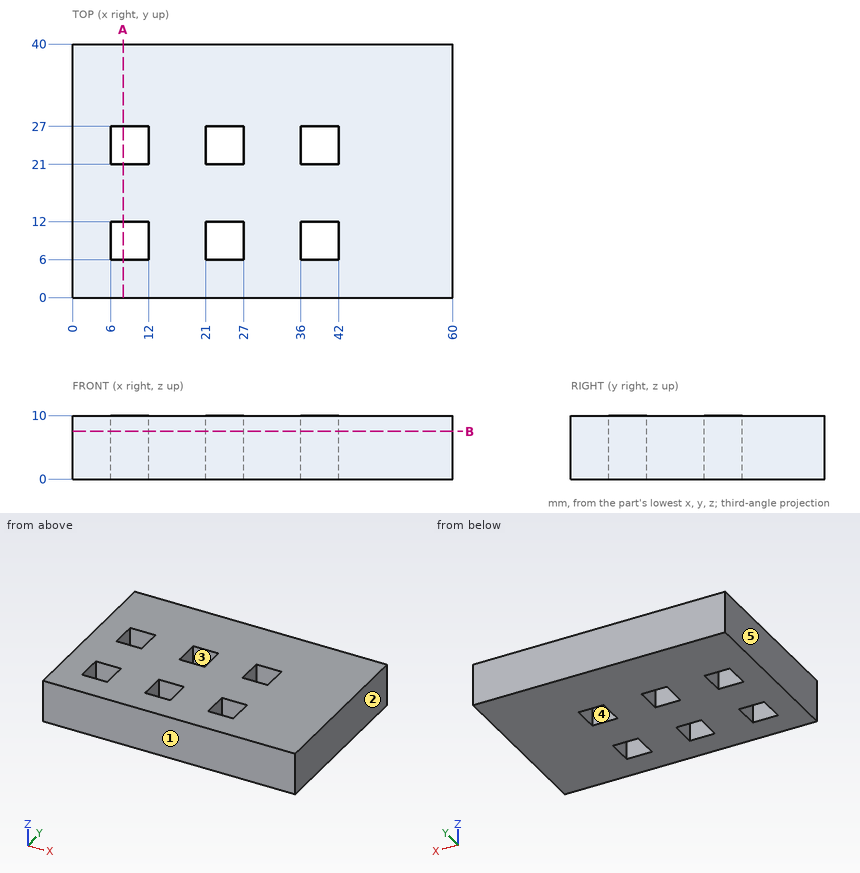
Geometry: see drawing. Coordinates: mm, zero at the bounding-box minimum. A direction names the side the tool comes from. Coordinates: 2 decimals unless noted, no trailing zeros. Loops run counter-clockwise (first coordinate to the right, second up) from the corner with the lowest first, then second, coordinate; pieces in that order, holes last. Notation, with made-up numbers: (-4.5, 75) - (42.5, 75) arc R20 cw to (42.5, 104) - close; hole circle Ø8 at (-33.75, 47). An arc over 180 degrees is marked (long way). Put each result on its own line as item: value. Start each with the question number.
Q1. Line query: line 1 (Y direction, x = 39, z = 7.25); line 2 (X direction, y = 10.5, z = 4.75). Output: solid intervals per line, ascending.
Q2. Cut plane A-A, the plane x = 8. Return loops of the section in (y, z), and give its area (3 significant figures).
Q3. Set-up query: the marked faces 4 and 5. Return all of +Z, -Z, +X, -X, +Y, -Y with unobstructed straight access to the full face (end or side cutting, diameter ignored); none if empty.
Q4. Cut plane B-B, the plane z = 7.5. Return loops of the section in (x, y).
Q5. Pull-direction query (Y, two-part tool) for the marked faces 1, 2 and 3; classes: released by +Y, released by -Y, zero draft, split by the parting line, or undercut.
Filled sheet:
1. line 1: 0 to 6, 12 to 21, 27 to 40
1. line 2: 0 to 6, 12 to 21, 27 to 36, 42 to 60
2. outline: (0, 0) - (6, 0) - (6, 10) - (0, 10) - close; (12, 0) - (21, 0) - (21, 10) - (12, 10) - close; (27, 0) - (40, 0) - (40, 10) - (27, 10) - close
2. area: 280 mm²
3. face 4: +Z, -Z
3. face 5: +Z, -Z, -X, +Y, -Y
4. outline: (0, 0) - (60, 0) - (60, 40) - (0, 40) - close; hole (6, 6) - (12, 6) - (12, 12) - (6, 12) - close; hole (6, 21) - (12, 21) - (12, 27) - (6, 27) - close; hole (21, 6) - (27, 6) - (27, 12) - (21, 12) - close; hole (21, 21) - (27, 21) - (27, 27) - (21, 27) - close; hole (36, 6) - (42, 6) - (42, 12) - (36, 12) - close; hole (36, 21) - (42, 21) - (42, 27) - (36, 27) - close
5. face 1: released by -Y
5. face 2: zero draft
5. face 3: undercut
